```python
from build123d import *

# Parameters (mm, degrees)
F0_W     = 30
F0_H     = 12
F1_DEPTH = 4
F2_W     = 15
F2_H     = 1
F3_DEPTH = 25
F5_D     = 1.7


with BuildPart() as f1:
    # F0 (on Top) → F1 (new body, symmetric)
    with BuildSketch(Plane.XY):
        Rectangle(F0_W, F0_H)
    extrude(amount=F1_DEPTH, both=True)

    # F2 (on face) → F3 (cut)
    with BuildSketch(Plane(origin=(0, 6, 0), x_dir=(-1, 0, 0), z_dir=(0, 1, 0))):
        with Locations((7.5, 3.5)):
            Rectangle(F2_W, F2_H)
    extrude(amount=-F3_DEPTH, mode=Mode.SUBTRACT)

    # F5 (through all)
    with Locations(Plane(origin=(0, 0, -4), x_dir=(1, 0, 0), z_dir=(0, 0, -1))):
        with Locations((-13, -3.5), (-13, 0), (-13, 3.5)):
            Hole(F5_D / 2)


solid = f1.part
```
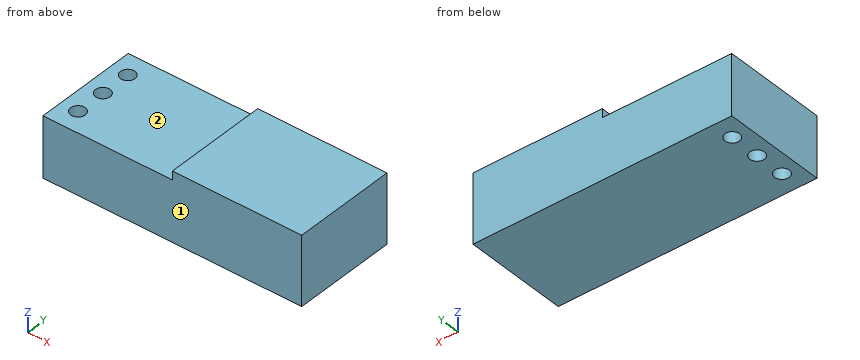
Part model, mm, in its own coordinate system. Face numbers are marked on the shaded views. A direction names the side the tool comes from. Give positions to 0.01 mm unless a question says otherwise; leave off trailing zeros. Order: outer loops, then holes, each group sorted by start corner. A loop starts at its lowest first (then second) coordinate and runs counter-clockwise, first axis right, second up. Notation, with made-up numbers: M 61.25,72 L 82.25,72 A36 cw 82.25,108 Z; hole C -23,51 d10. An arc over 180 degrees is marked long. Use a Markdown table: item, result. Add a question column.
(1) Saw through at C-C, the plane z = -0.75. Give the cut face in (x, y).
(2) Saw through at D-D, the plane y = 5. Give the cut face in (x, z).
(3) Drop flat-ended pins along their axis: P1, Ø2.5, axis at x = -13, y = 3.5, coming from the +Z side; P2, Ø0.5, axis at y = -2, z = 3.5, coming from the -X side. Give the stop position or say it passes through.
(4) Probe line 1 along Y through (x, z) = (-13, 2.5); line 2 along X through (y, z) = (3.5, -2.25); line 3 along X through (y, z) = (4.25, -2.75). List the from-to ranges inside material, lowest first. Write a range as [from, to].
(5) Saw through at B-B, the plane x = -13. Give the cut face in (y, z).
(6) Saw through at A-A, the plane y = -3.5. Give the cut face in (x, z).
(7) 3-axis set-ups, long thin cutter, end or side, ignore diameter. For the marked faces 1 and 2: which of +Z, -Z, +X, -X, +Y, -Y reach the whole face in a straight line?
Answer key:
| question | item | result |
|---|---|---|
| 1 | outline | M -15,-6 L 15,-6 L 15,6 L -15,6 Z; hole C -13,-3.5 d1.7; hole C -13,0 d1.7; hole C -13,3.5 d1.7 |
| 2 | outline | M -15,-4 L 15,-4 L 15,4 L 0,4 L 0,3 L -15,3 Z |
| 3 | P1 | z = 3 |
| 3 | P2 | x = 0 |
| 4 | line 1 | [-6, -4.35], [-2.65, -0.85], [0.85, 2.65], [4.35, 6] |
| 4 | line 2 | [-15, -13.85], [-12.15, 15] |
| 4 | line 3 | [-15, -13.4], [-12.6, 15] |
| 5 | outline | M -6,-4 L -4.35,-4 L -4.35,3 L -6,3 Z; M -2.65,-4 L -0.85,-4 L -0.85,3 L -2.65,3 Z; M 0.85,-4 L 2.65,-4 L 2.65,3 L 0.85,3 Z; M 4.35,-4 L 6,-4 L 6,3 L 4.35,3 Z |
| 6 | outline | M -15,-4 L -13.85,-4 L -13.85,3 L -15,3 Z; M -12.15,-4 L 15,-4 L 15,4 L 0,4 L 0,3 L -12.15,3 Z |
| 7 | face 1 | +Z, -Z, +X, -X, -Y |
| 7 | face 2 | +Z, -X, +Y, -Y |
